from build123d import *

# Parameters (mm, degrees)
F0_R     = 25
F0_R_2   = 3.5
F1_DEPTH = 18.5
F2_R     = 7.5
F2_R_2   = 3.5
F3_DEPTH = 2.6
F4_R     = 17.8
F4_R_2   = 15
F5_DEPTH = 3
F6_SIZE2 = 0.5
F6_SIZE  = 0.5
F7_SIZE  = 1.5


with BuildPart() as f1:
    # F0 (on Front) → F1 (new body)
    with BuildSketch(Plane.XZ):
        Circle(F0_R)
        Circle(F0_R_2, mode=Mode.SUBTRACT)
    extrude(amount=F1_DEPTH)

    # F2 (on face) → F3 (join)
    with BuildSketch(Plane.XZ.offset(18.5)):
        Circle(F2_R)
        Circle(F2_R_2, mode=Mode.SUBTRACT)
    extrude(amount=F3_DEPTH)

    # F4 (on face) → F5 (cut)
    with BuildSketch(Plane(origin=(0, 0, 0), x_dir=(-1, 0, 0), z_dir=(0, 1, 0))):
        Circle(F4_R)
        Circle(F4_R_2, mode=Mode.SUBTRACT)
    extrude(amount=-F5_DEPTH, mode=Mode.SUBTRACT)

    # F6
    f6_edges = [f1.edges().sort_by_distance(p)[0] for p in [
        (-25, 0, 0),
        (-25, -18.5, 0),
        (-3.5, 0, 0),
        (-7.5, -21.1, 0),
    ]]
    chamfer(f6_edges, length=F6_SIZE, length2=F6_SIZE2)

    # F7
    f7_edges = [f1.edges().sort_by_distance(p)[0] for p in [
        (-3.5, -21.1, 0),
    ]]
    chamfer(f7_edges, length=F7_SIZE)


solid = f1.part
Can you work these out from the model? Positions are in its coordinate system, mm. A direction names the side the tool comes from. Give positions to 0.01 mm unless a question says otherwise; leave off trailing zeros. Order: outer loops, then holes, each group sorted by start corner. A loop starts at its lowest first (then second) coordinate and runs counter-clockwise, first axis right, second up. Notation, with made-up numbers: M -8,-37 L 25,-37 A24 ccw 25,-5 Z; hole C -23.5,-12 d11. An arc over 180 degrees is marked long. Use a Markdown table: item, result. Add a question column.
Item 1: We'd pull the mould along X, two halves only. Please class faces 1 (the cylindrical face through (14.985, -1.479, 0.66)), 2 (the cylindrical face through (-7.493, -19.535, 0.33)), 3 (the flat face through (3, 0, -3)): +X half, -X half, draft (parallel to the pull), parting line (faces both ways), or undercut.
Item 2: If I drill on L1, parallel to Z at x = 0, y = -1.55; L2, parallel to Z at x = 0, y = -10.5; L3, parallel to Y at x = 0, z = 20.5, over which ranges is the centre line in solid material (lowest first)? Write a range as [from, to].
Item 3: Suppose I cut it at C-C (y = -14). List the corners of the cut face in (x, z) for me, then the cut area to 3 significant figures.
Item 4: Will these pins go through, and if not, where does the flat tip stop? pin 1 (1 mm diameter, centred on x = -5, z = -17.5, fed in from -Y); pin 2 (9 mm diameter, centred on x = 0, z = 0, fed in from +Y); pin 3 (6 mm diameter, centred on x = 13.5, y = -13, fed in from +Z); pin 4 (1 mm diameter, centred on x = -15, y = -2, fed in from +Z).
Item 5: For faces 4 (the flat face through (8, -3, -13)), 5 (the flat face through (5, -18.5, 6)), 6 (the flat face through (13, 0, 13)), which set-ups out of +Z, -Z, +X, -X, +Y, -Y let a thin tool reach every point of the face, with its end or its side?
Answer sheet:
| question | item | result |
|---|---|---|
| 1 | face 1 | undercut |
| 1 | face 2 | parting line |
| 1 | face 3 | draft |
| 2 | L1 | z = [-25, -17.8], [-15, -3.5], [3.5, 15], [17.8, 25] |
| 2 | L2 | z = [-25, -3.5], [3.5, 25] |
| 2 | L3 | y = [-18.5, 0] |
| 3 | outline | C 0,0 d50; hole C 0,0 d7 |
| 3 | area | 1,930 mm² |
| 4 | pin 1 | stops at y = -18.5 |
| 4 | pin 2 | stops at y = 0 |
| 4 | pin 3 | stops at z = 22.69 |
| 4 | pin 4 | stops at z = 20.37 |
| 5 | face 4 | +Y |
| 5 | face 5 | -Y |
| 5 | face 6 | +Z, -Z, +X, -X, +Y |
